Read the model definition and answer for the solid it produces. Units are mm, in the model's axes. Give positions to 0.01 mm unless a question says otherwise; leave off trailing zeros. Order: outer loops, then holes, each group sorted by start corner. A loop starts at its lowest first (then second) coordinate and runs counter-clockwise, first axis right, second up.
Item 1: Given pin 1 Ø0.6 at (x, y) = (24.5, -2) entering from +Z; pin 2 Ø0.6 at (x, z) = (24, 0.5) entering from +Y; pin 3 Ø1 at (x, z) = (24, 0.5) entering from -Y, each flat-ended and moving along its own axis, determine where each tip first touches the part or whether it passes through.
Item 2: A cutting plane is placed at A-A (z = 1.05). Write down the section's boundary in (x, y), plus the area to 3 significant figures.
Item 3: Find the intervals of material crossed by line 1 along X through (y, z) = (-1.45, -1.15); line 2 along X through (y, z) = (-4.75, 2.05), in increasing order.
Item 4: A cutting plane is placed at B-B (y = -2.85). Write down the section's boundary in (x, z).
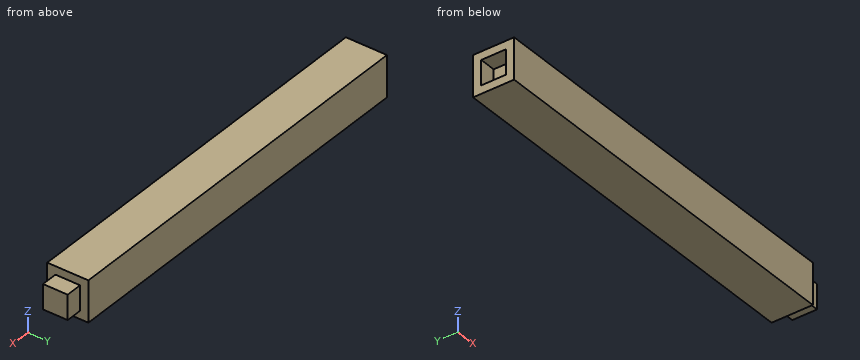
from build123d import *

# Parameters (mm, degrees)
F0_W     = 50
F0_H     = 5
F1_DEPTH = 5
F2_W     = 3
F2_H     = 3
F3_DEPTH = 2
F4_W     = 5
F4_H     = 5
F4_W_2   = 3
F4_H_2   = 3
F5_DEPTH = 2


with BuildPart() as f1:
    # F0 (on Front) → F1 (new body)
    with BuildSketch(Plane.XZ):
        Rectangle(F0_W, F0_H)
    extrude(amount=F1_DEPTH)

    # F2 (on face) → F3 (cut)
    with BuildSketch(Plane(origin=(-25, 0, 0), x_dir=(0, -1, 0), z_dir=(-1, 0, 0))):
        with Locations((2.5, 0)):
            Rectangle(F2_W, F2_H)
    extrude(amount=-F3_DEPTH, mode=Mode.SUBTRACT)

    # F4 (on face) → F5 (cut)
    with BuildSketch(Plane.YZ.offset(25)):
        with Locations((-2.5, 0)):
            Rectangle(F4_W, F4_H)
        with Locations((-2.5, 0)):
            Rectangle(F4_W_2, F4_H_2, mode=Mode.SUBTRACT)
    extrude(amount=-F5_DEPTH, mode=Mode.SUBTRACT)


solid = f1.part
Response values:
1. pin 1: stops at z = 1.5
1. pin 2: stops at y = -1
1. pin 3: stops at y = -4
2. outline: (-25, -5) - (23, -5) - (23, -4) - (25, -4) - (25, -1) - (23, -1) - (23, 0) - (-25, 0) - (-25, -1) - (-23, -1) - (-23, -4) - (-25, -4) - close
2. area: 240 mm2
3. line 1: x = -23 to 25
3. line 2: x = -25 to 23
4. outline: (-25, -2.5) - (23, -2.5) - (23, -1.5) - (25, -1.5) - (25, 1.5) - (23, 1.5) - (23, 2.5) - (-25, 2.5) - (-25, 1.5) - (-23, 1.5) - (-23, -1.5) - (-25, -1.5) - close
